from build123d import *

# Parameters (mm, degrees)
SKETCH_1_W          = 350
SKETCH_1_H          = 350
EXTRUDE_1_DEPTH     = 100
FILLET_1_R          = 50
CUT_EXTRUDE_1_DEPTH = 35
SKETCH_4_W          = 75
SKETCH_4_H          = 130
CUT_EXTRUDE_2_DEPTH = 75
EXTRUDE_3_REACH     = 388.685
SKETCH_5_R          = 10
FILLET_2_R          = 10
CUT_EXTRUDE_3_DEPTH = 75
SKETCH_7_R          = 10
SKETCH_7_R_2        = 4
EXTRUDE_4_DEPTH     = 38.62
SKETCH_8_W          = 75
SKETCH_8_H          = 150
EXTRUDE_5_DEPTH     = 75
FILLET_3_R          = 30
SKETCH_9_R          = 10
EXTRUDE_6_DEPTH     = 5


with BuildPart() as part:
    # 草图1 → 凸台-拉伸1 (new body)
    with BuildSketch(Plane.XY):
        Rectangle(SKETCH_1_W, SKETCH_1_H)
    extrude(amount=EXTRUDE_1_DEPTH)

    # 圆角1
    fillet_1_edges = [part.edges().sort_by_distance(p)[0] for p in [
        (-175, 175, 50),
        (175, 175, 50),
        (175, -175, 50),
        (-175, -175, 50),
    ]]
    fillet(fillet_1_edges, radius=FILLET_1_R)

    # 草图3 → 切除-拉伸1 (cut, symmetric)
    with BuildSketch(Plane.ZY.offset(120)):
        with BuildLine():
            Line((15, 75.934955472), (100, 75.934955472))
            Line((100, 75.934955472), (100, 140.934955472))
            Line((100, 140.934955472), (80, 140.934955472))
            ThreePointArc((80, 140.934955472), (34.038059223, 121.896896249), (15, 75.934955472))
        make_face()
        with BuildLine():
            Line((100, 10.934955472), (100, 75.934955472))
            Line((100, 75.934955472), (15, 75.934955472))
            ThreePointArc((15, 75.934955472), (34.038059223, 29.973014695), (80, 10.934955472))
            Line((80, 10.934955472), (100, 10.934955472))
        make_face()
    cut_extrude_1 = extrude(amount=CUT_EXTRUDE_1_DEPTH, both=True, mode=Mode.SUBTRACT)

    # 镜向1: 切除-拉伸1 across plane
    add(cut_extrude_1.mirror(Plane(origin=(0, 0, 0), x_dir=(0, 0, 1), z_dir=(1, 0, 0))), mode=Mode.SUBTRACT)

    # 草图4 → 切除-拉伸2 (cut)
    with BuildSketch(Plane.XY.offset(100)):
        with Locations((0, 75.934955472)):
            Rectangle(SKETCH_4_W, SKETCH_4_H)
    extrude(amount=-CUT_EXTRUDE_2_DEPTH, mode=Mode.SUBTRACT)

    # 凸台-拉伸3: up to this face of the body (flat: up to its plane)
    extrude_3_end = Plane(part.part.faces().sort_by_distance((155, 75.934955472, 62.993408065))[0])
    # 草图5 → 凸台-拉伸3 (add, up to the picked face)
    with BuildSketch(Plane(origin=(-155, 0, 0), x_dir=(0, 0, -1), z_dir=(1, 0, 0)), mode=Mode.PRIVATE) as extrude_3_sk1:
        with Locations(Location((-90, 75.934955472, 0), (0, 0, 180))):
            Circle(SKETCH_5_R)
    extrude_3_tool1 = split(extrude(extrude_3_sk1.sketch, amount=EXTRUDE_3_REACH, mode=Mode.PRIVATE), bisect_by=extrude_3_end, keep=Keep.BOTH, mode=Mode.PRIVATE)
    add(extrude_3_tool1.solids().sort_by(Axis((-155, 75.934955, 90), (1, 0, 0)))[0])

    # 圆角2
    fillet_2_edges = [part.edges().sort_by_distance(p)[0] for p in [
        (-120, 10.934955472, 100),
        (-120, 140.934955472, 100),
        (120, 140.934955472, 100),
        (120, 10.934955472, 100),
    ]]
    fillet(fillet_2_edges, radius=FILLET_2_R)

    # 草图6 → 切除-拉伸3 (cut)
    with BuildSketch(Plane.XY.offset(100)):
        with BuildLine():
            Line((170, -20), (0, -20))
            Line((0, -20), (0, -170))
            Line((0, -170), (125, -170))
            ThreePointArc((125, -170), (156.819805153, -156.819805153), (170, -125))
            Line((170, -125), (170, -20))
        make_face()
        with BuildLine():
            Line((0, -170), (0, -20))
            Line((0, -20), (-170, -20))
            Line((-170, -20), (-170, -125))
            ThreePointArc((-170, -125), (-156.819805153, -156.819805153), (-125, -170))
            Line((-125, -170), (0, -170))
        make_face()
    extrude(amount=-CUT_EXTRUDE_3_DEPTH, mode=Mode.SUBTRACT)

    # 草图7 → 凸台-拉伸4 (add)
    # profile 1 of 2: a face of its own
    with BuildSketch(Plane.XY.offset(25)):
        with Locations(Location((110, -110, 0), (0, 0, 180))):
            Circle(SKETCH_7_R)
        with Locations(Location((110, -110, 0), (0, 0, 180))):
            Circle(SKETCH_7_R_2, mode=Mode.SUBTRACT)
    # profile 2 of 2: a face of its own
    with BuildSketch(Plane.XY.offset(25)):
        with Locations(Location((-110, -110, 0), (0, 0, 180))):
            Circle(SKETCH_7_R)
        with Locations(Location((-110, -110, 0), (0, 0, 180))):
            Circle(SKETCH_7_R_2, mode=Mode.SUBTRACT)
    extrude(amount=EXTRUDE_4_DEPTH)

    # 草图8 → 凸台-拉伸5 (add)
    with BuildSketch(Plane.XY.offset(25)):
        with Locations((0, -95)):
            Rectangle(SKETCH_8_W, SKETCH_8_H)
    extrude(amount=EXTRUDE_5_DEPTH)

    # 圆角3
    fillet_3_edges = [part.edges().sort_by_distance(p)[0] for p in [
        (-170, -20, 62.5),
        (170, -20, 62.5),
        (-37.5, -170, 62.5),
        (37.5, -170, 62.5),
        (37.5, -20, 62.5),
        (-37.5, -20, 62.5),
    ]]
    fillet(fillet_3_edges, radius=FILLET_3_R)

    # 草图9 → 凸台-拉伸6 (add)
    with BuildSketch(Plane(origin=(0, 175, 0), x_dir=(1, 0, 0), z_dir=(0, 1, 0))):
        with Locations((-73.626122366, -34.222973779)):
            Circle(SKETCH_9_R)
        with Locations((73.626122366, -34.222973779)):
            Circle(SKETCH_9_R)
    extrude(amount=EXTRUDE_6_DEPTH)


solid = part.part
Can you work these out from the model? Positions are in its coordinate system, mm. A direction names the side the tool comes from. Coordinates: 2 decimals unless noted, no trailing zeros. Write each loop counter-clockwise with the first axis right and the second up, starting at its lowest first coordinate (ties: lowest second). Pieces come first, ordered by that corner, then holes. Notation, with made-up numbers: (83.5, -22) - (133.5, -22) arc R14 ccw to (133.5, 1) - close; hole circle Ø2 at (82.25, 43.25). An arc over 180 degrees is marked (long way). Return JSON: item names as keys, results as strings. Group by question number.
Item 1: Please list where these lines run through material, in increasing order: probe 1 along X at (y, z) = (97.5, 62); probe 2 along Y at (x, z) = (-112, 57.5); probe 3 along Y at (x, z) = (-3.5, 77).
Item 2: Which directions (+Z, -Z, +X, -X, +Y, -Y) give clear straight access to the entire face, cutting with the end or side of a thin tool? Please do faces 1 (the face through (-37.5, -96, 62)), 2 (the face through (-0.525, 82.02, 82.064)), 3 (the face through (-2, 2, 0)).
Item 3: We'd pull the mould along X, two halves only. Please class faces 4 (the face through (-119.51, 143.942, 97.148)), 5 (the face through (175, -2, 49)), 6 (the face through (-74, 180, 34)), 7 (the face through (82.864, 177.465, 38.053)): pulls with the +X half, pulls with the -X half, needs draft (parallel to the pull), parting line crosses it, or undercut.
Item 4: I'm going to push flat-ended pins straight in: pin 1 Ø6 at (x, z) = (98, 49.5) entering from +Y; pin 2 Ø22.5 at (x, y) = (2.5, 108) entering from +Z; pin 3 Ø10 at (x, y) = (-98.5, 122.5) entering from +Z. Where does each tip first touch, or does it pass through?
Item 5: If we section it at A-A (x = -43): Write out the boundary of the cut face in (y, z).
Return value:
{
 "1": {"probe 1": "x = -175 to -155, -85 to -37.5, 37.5 to 85, 155 to 175", "probe 2": "y = -175 to -170, -119.8 to -113.46, -106.54 to -100.2, -20 to 14.95, 136.92 to 175", "probe 3": "y = -175 to 10.93, 140.93 to 175"},
 "2": {"face 1": "+Z", "face 2": "none", "face 3": "-Z, +X, -X, +Y, -Y"},
 "3": {"face 4": "undercut", "face 5": "pulls with the +X half", "face 6": "needs draft", "face 7": "undercut"},
 "4": {"pin 1": "stops at y = 175", "pin 2": "stops at z = 25", "pin 3": "stops at z = 40.43"},
 "5": {"outline": "(-175, 0) - (175, 0) - (175, 100) - (-32.69, 100) - (-32.69, 25) - (-157.31, 25) - (-157.31, 100) - (-175, 100) - close"}
}
